Build history of the part. All positions in model axes, mm. Face numbers are marked on the shaded views. A direction names the side the tool comes from. Round coordinates to 2 decimals unless told otherwise and drop trailing zeros. Loops run counter-clockwise (first coordinate to the right, second up) from the corner with the lowest first, then second, coordinate; pieces in that order, holes last.
from build123d import *

# Parameters (mm, degrees)
F0_W      = 71.12
F0_H      = 50.8
F1_DEPTH  = 76.2
F3_T      = -2.54
F4_DEPTH  = 50.8
F5_DEPTH  = 50.8
F7_DEPTH  = 12.7
F8_DEPTH  = 12.7
F9_DEPTH  = 12.7
F12_DEPTH = 5.08
F13_DEPTH = 5.08


with BuildPart() as f1:
    # F0 (on Top) → F1 (new body)
    with BuildSketch(Plane.XY):
        with Locations((-1.6881457889, -10.255297339)):
            Rectangle(F0_W, F0_H)
    extrude(amount=F1_DEPTH)

    # F3
    f3_openings = [f1.faces().sort_by_distance(p)[0] for p in [
        (-1.688146, -35.655297, 38.1),
    ]]
    offset(amount=F3_T, openings=f3_openings)

    # F2 (on face) → F4 (join)
    with BuildSketch(Plane.XZ.offset(35.655297339)):
        Polygon((-37.2481457889, 49.53), (-37.2481457889, 46.99), (-1.6881457889, 46.99), (33.8718542111, 46.99), (33.8718542111, 49.53), align=None)
    extrude(amount=-F4_DEPTH)

    # F2 (on face) → F5 (join)
    with BuildSketch(Plane.XZ.offset(35.655297339)):
        Polygon((-37.2481457889, 19.05), (-1.6881457889, 19.05), (33.8718542111, 19.05), (33.8718542111, 21.59), (-1.6881457889, 21.59), (-37.2481457889, 21.59), align=None)
    extrude(amount=-F5_DEPTH)

    # F6 (on face) → F7 (join)
    with BuildSketch(Plane(origin=(-37.2481457889, 0, 0), x_dir=(0, -1, 0), z_dir=(-1, 0, 0))):
        with BuildLine():
            ThreePointArc((11.842797339, 73.66), (9.1327653238, 74.7825320151), (10.255297339, 72.0725))
            ThreePointArc((10.255297339, 72.0725), (11.3778293541, 72.5374679849), (11.842797339, 73.66))
        make_face()
    extrude(amount=F7_DEPTH)

    # F6 (on face) → F8 (join)
    with BuildSketch(Plane(origin=(-37.2481457889, 0, 0), x_dir=(0, -1, 0), z_dir=(-1, 0, 0))):
        with BuildLine():
            Line((22.955297339, 63.5), (22.955297339, 61.9125))
            ThreePointArc((22.955297339, 61.9125), (24.0778293541, 62.3774679849), (24.542797339, 63.5))
            ThreePointArc((24.542797339, 63.5), (22.955297339, 65.0875), (21.367797339, 63.5))
            Line((21.367797339, 63.5), (22.955297339, 63.5))
        make_face()
    extrude(amount=F8_DEPTH)

    # F6 (on face) → F9 (join)
    with BuildSketch(Plane(origin=(-37.2481457889, 0, 0), x_dir=(0, -1, 0), z_dir=(-1, 0, 0))):
        with BuildLine():
            ThreePointArc((21.367797339, 63.5), (21.8327653238, 62.3774679849), (22.955297339, 61.9125))
            Line((22.955297339, 61.9125), (22.955297339, 63.5))
            Line((22.955297339, 63.5), (21.367797339, 63.5))
        make_face()
    extrude(amount=F9_DEPTH)

    # F11: F1 across plane


with BuildPart() as f1_1:
    add(f1.part)
    add(f1.part.mirror(Plane.YZ.offset(-2.54)))

    # F12 (add): a face of the model
    f12_faces = [f1_1.faces().sort_by_distance(p)[0] for p in [
        (-38.9518542111, -10.2292152391, 37.9748059207),
    ]]
    extrude(f12_faces, amount=F12_DEPTH)

    # F13 (add): a face of the model
    f13_faces = [f1_1.faces().sort_by_distance(p)[0] for p in [
        (33.8718542111, -10.2292152391, 37.9748059207),
    ]]
    extrude(f13_faces, amount=F13_DEPTH)


solid = f1_1.part
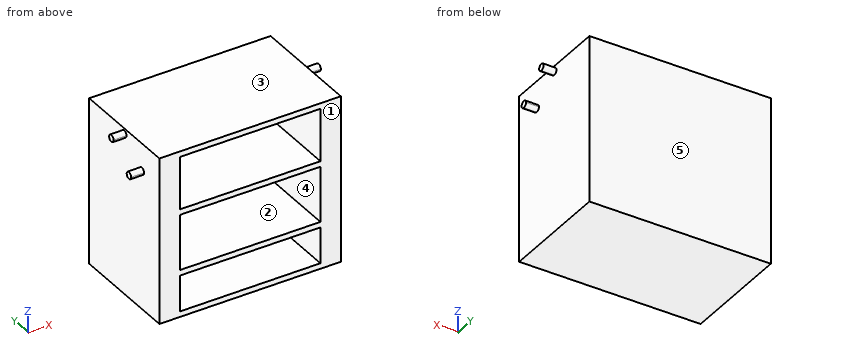
(1) Probe line 1 (Z direction, x = -2, y = -22.5); line 2 (X direction, y = -26, z = 13.5); line 3 (X direction, y = -11, z = 73). List the from-to ranges inside material, lowest first.
Responses:
line 1: z = 0 to 2.54, 19.05 to 21.59, 46.99 to 49.53, 73.66 to 76.2
line 2: x = -44.03 to -34.71, 29.63 to 38.95
line 3: x = -49.95 to -34.71, 29.63 to 44.87
(2) Slice it at A-A on z = 11.5. List the corners of the cut face in (x, y).
Responses:
outline: (-44.03, -35.66) - (-34.71, -35.66) - (-34.71, 12.6) - (29.63, 12.6) - (29.63, -35.66) - (38.95, -35.66) - (38.95, 15.14) - (-44.03, 15.14) - close
(3) Pin check, flat tips, straight feed: P1, Ø2, axis at y = -28, z = 8.5, coming from the -X side; P2, Ø20.5, axis at y = -21, z = 29.5, coming from the +X side; P3, Ø12.5, axis at x = 4.5, z = 38, coming from the -Y side. Stop position of each tip, or through.
Responses:
P1: stops at x = -44.03
P2: stops at x = 38.95
P3: stops at y = 12.6
(4) Slice it at B-B on y = 5.5. List the corners of the cut face in (x, z), plus the area to 3 significant figures.
Responses:
outline: (-44.03, 0) - (38.95, 0) - (38.95, 76.2) - (-44.03, 76.2) - close; hole (-34.71, 2.54) - (29.63, 2.54) - (29.63, 19.05) - (-34.71, 19.05) - close; hole (-34.71, 21.59) - (29.63, 21.59) - (29.63, 46.99) - (-34.71, 46.99) - close; hole (-34.71, 49.53) - (29.63, 49.53) - (29.63, 73.66) - (-34.71, 73.66) - close
area: 2,070 mm2
(5) Which spindle directions (+Z, -Z, +X, -X, +Y, -Y) get a long thin tool onto all of the face, cutting with end or side? Do the marked faces 1 and 2. Say none if no direction does.
Responses:
face 1: +Z, -Z, +X, -X, -Y
face 2: -Y
(6) Slice it at C-C on x = -22.5. List the corners of the cut face in (y, z), plus the area to 3 significant figures.
Responses:
outline: (-35.66, 0) - (15.14, 0) - (15.14, 76.2) - (-35.66, 76.2) - (-35.66, 73.66) - (12.6, 73.66) - (12.6, 49.53) - (-35.66, 49.53) - (-35.66, 46.99) - (12.6, 46.99) - (12.6, 21.59) - (-35.66, 21.59) - (-35.66, 19.05) - (12.6, 19.05) - (12.6, 2.54) - (-35.66, 2.54) - close
area: 684 mm2
(7) Pull direction Z, two halves, no side cores. Call the marked faces 3, 4 and 5: +Z half, -Z half, draft (parallel to the pull), parting line (faces both ways), or undercut.
Responses:
face 3: +Z half
face 4: undercut
face 5: draft
